Source: CAD feature listing. Evaluate the final solid. Frame: model axes, mm. A direction names the side the tool comes from. Round coordinates to 2 decimals unless told otherwise and drop trailing zeros. Order: outer loops, then holes, each group sorted by start corner. A loop starts at its lowest first (then second) coordinate and runs counter-clockwise, first axis right, second up. Notation, with made-up numbers: (-18.75, 82.25) - (34.25, 82.25) arc R20 cw to (34.25, 98.25) - close; hole circle Ø6 at (-38.75, -8). An arc over 180 degrees is marked (long way). Put each result on its own line as item: value. Start each with the question number.
1) Section D-D on x = 2.35. Output: boundary loops of the cut face in (y, z), then the cut area to 3 significant figures.
2) Section B-B on y = -3.5. Output: boundary loops of the cut face in (x, z).
3) Section A-A on y = 3. Output: boundary loops of the cut face in (x, z).
4) Mould query, pull axis Y, two halves, no side actions, for faces 1 (the face through (-3.3, 0.6, 2.5)), 2 (the face through (5, 3, 2)), 3 (the face through (-1.98, 2.29, 2.46)). Classes: +Y half, -Y half, draft (parallel to the pull), parting line (faces both ways), or undercut.
5) Section C-C on z = 1.4. Output: boundary loops of the cut face in (x, y), then the cut area to 3 significant figures.
6) Access query for faces 4 (the face through (3.3, 0.6, 2.5)), 5 (the face through (0, 6.5, 2)), 6 (the face through (-1.444, 5.021, 2.215)). Directions: +Z, -Z, +X, -X, +Y, -Y. A direction counts if a zero-diameter tool reaches every point of the face in a straight line with its end or side. Return the directions, or none.
7) Contact query for flat-ended pins moving along their axis: P1, Ø3, axis at x = 2.35, z = 2.5, coming from the -Y side; P2, Ø2.5, axis at y = -4, z = 2.5, coming from the +X side; P3, Ø1.1, axis at x = -2.35, z = 2.5, coming from the -Y side; P4, Ø2.5, axis at y = -4.5, z = 1.5, coming from the -X side. Output: stop coordinate, or through.
8) Line query: probe 1 along X at (y, z) = (5.5, 2.55); probe 2 along Z at (x, y) = (2.35, 5.2); probe 3 along X at (y, z) = (-0.25, 2.75). Output: solid intervals per line, ascending. Write a range as [from, to].
```python
from build123d import *

# Parameters (mm, degrees)
SKETCH1_W           = 10
SKETCH1_H           = 13
SKETCH1_R           = 0.8
BOSS_EXTRUDE1_DEPTH = 5
CUT_EXTRUDE2_DEPTH  = 3.5
SKETCH4_R           = 1.25
CUT_EXTRUDE3_DEPTH  = 7.5
SKETCH5_R           = 0.95
CUT_EXTRUDE4_DEPTH  = 3


with BuildPart() as part:
    # Sketch1 → Boss-Extrude1 (new body)
    with BuildSketch(Plane.XY):
        Rectangle(SKETCH1_W, SKETCH1_H)
        with Locations((-2.35, 3)):
            Circle(SKETCH1_R, mode=Mode.SUBTRACT)
        with Locations((2.35, 3)):
            Circle(SKETCH1_R, mode=Mode.SUBTRACT)
    extrude(amount=BOSS_EXTRUDE1_DEPTH)

    # Sketch3 → Cut-Extrude2 (cut)
    with BuildSketch(Plane.ZY.offset(5)):
        with BuildLine():
            Line((-1.6, -3.5), (-1.6, -7.6))
            Line((-1.6, -7.6), (6.6, -7.6))
            Line((6.6, -7.6), (6.6, -3.5))
            ThreePointArc((6.6, -3.5), (2.5, 0.6), (-1.6, -3.5))
        make_face()
    cut_extrude2 = extrude(amount=-CUT_EXTRUDE2_DEPTH, mode=Mode.SUBTRACT)

    # Mirror1: Cut-Extrude2 across plane
    add(cut_extrude2.mirror(Plane(origin=(0, 0, 0), x_dir=(0, 0, 1), z_dir=(1, 0, 0))), mode=Mode.SUBTRACT)

    # Sketch4 → Cut-Extrude3 (cut, through all)
    with BuildSketch(Plane.ZY.offset(1.5)):
        with Locations((2.5, -3.5)):
            Circle(SKETCH4_R)
    extrude(amount=-CUT_EXTRUDE3_DEPTH, mode=Mode.SUBTRACT)

    # Sketch5 → Cut-Extrude4 (cut)
    with BuildSketch(Plane(origin=(0, 6.5, 0), x_dir=(1, 0, 0), z_dir=(0, 1, 0))):
        with Locations((-2.35, -2.5)):
            Circle(SKETCH5_R)
        with Locations((2.35, -2.5)):
            Circle(SKETCH5_R)
    extrude(amount=-CUT_EXTRUDE4_DEPTH, mode=Mode.SUBTRACT)


solid = part.part
```
Answer sheet:
1. outline: (-0.25, 0) - (2.2, 0) - (2.2, 5) - (-0.25, 5) arc R4.1 cw to start; (3.8, 0) - (6.5, 0) - (6.5, 1.55) - (3.8, 1.55) - close; (3.8, 3.45) - (6.5, 3.45) - (6.5, 5) - (3.8, 5) - close
1. area: 17.7 mm^2
2. outline: (-1.5, 0) - (1.5, 0) - (1.5, 1.25) - (-1.5, 1.25) - close; (-1.5, 3.75) - (1.5, 3.75) - (1.5, 5) - (-1.5, 5) - close
3. outline: (-5, 0) - (-3.15, 0) - (-3.15, 5) - (-5, 5) - close; (-1.55, 0) - (1.55, 0) - (1.55, 5) - (-1.55, 5) - close; (3.15, 0) - (5, 0) - (5, 5) - (3.15, 5) - close
4. face 1: -Y half
4. face 2: draft
4. face 3: undercut
5. outline: (-5, 0.45) - (-1.5, 0.45) - (-1.5, -2.91) - (1.5, -2.91) - (1.5, 0.45) - (5, 0.45) - (5, 6.5) - (-5, 6.5) - close; (-1.5, -6.5) - (1.5, -6.5) - (1.5, -4.09) - (-1.5, -4.09) - close; hole circle Ø1.6 at (-2.35, 3); hole circle Ø1.6 at (2.35, 3)
5. area: 73.8 mm^2
6. face 4: +X, -Y
6. face 5: +Z, -Z, +X, -X, +Y
6. face 6: +Y
7. P1: y = -6.5
7. P2: x = 1.5
7. P3: y = 0.56
7. P4: x = -1.5
8. probe 1: [-5, -3.3], [-1.4, 1.4], [3.3, 5]
8. probe 2: [0, 1.55], [3.45, 5]
8. probe 3: [-1.5, 1.5]
